Print and shaded views of the part. All mm, measured from the part's lowest x, y and z. A direction names the side the tool comes from. Round coordinates to 2 decimals unless told otherwise and drop trailing zeros. Write each loop counter-clockwise with the first axis right and the second up, starting at its lowest first coordinate (ties: lowest second). Pieces come first, ordered by that corner, then holes. Notation, with made-up numbers: (42, -30.75) - (77, -30.75) arc R13 cw to (77, -9.75) - close; hole circle Ø2 at (60.5, 6.25). An arc over 180 degrees is marked (long way). Answer as a JSON object with one key per item and string values. Group by question number.
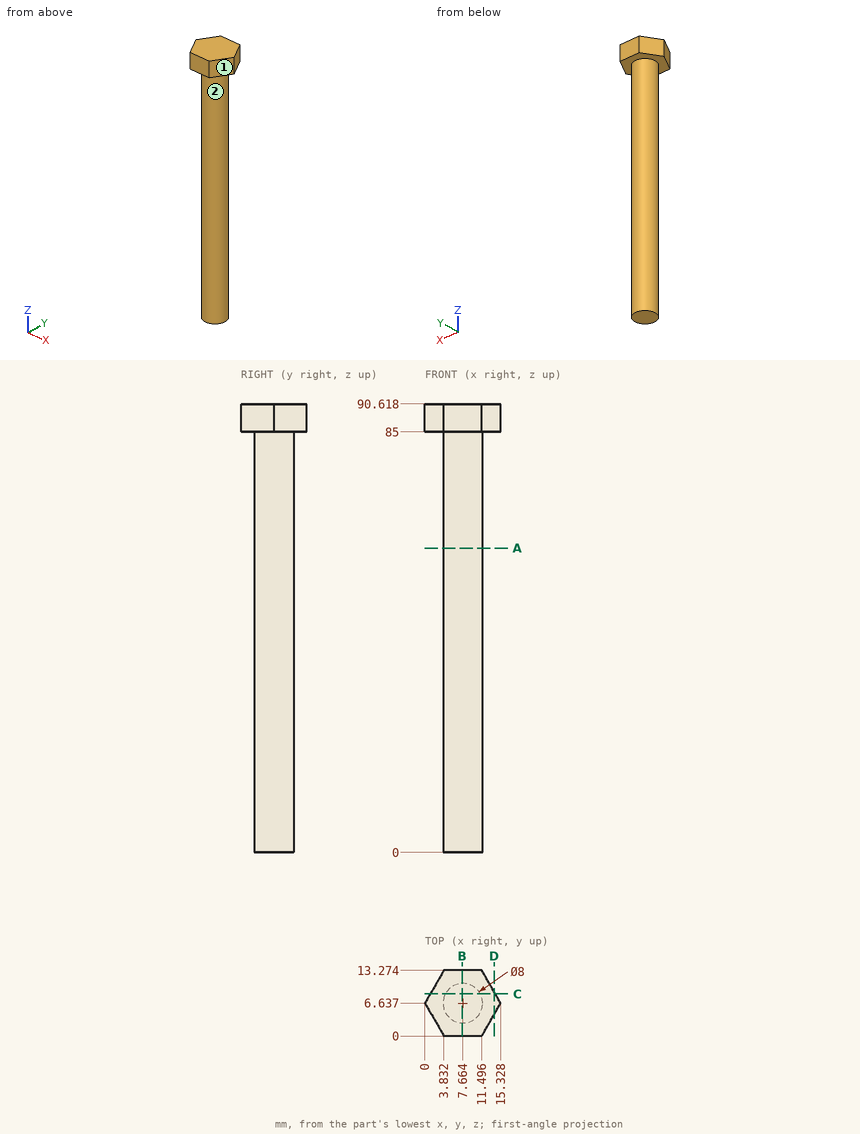
(1) 3-axis set-ups, long thin cutter, end or side, ignore diameter. For the marked faces 1 and 2: which of +Z, -Z, +X, -X, +Y, -Y reach the whole face in a straight line?
(2) Flat gauge pins, fed straight in: pin 1 (4 mm diameter, centred on x = 11, z = 34.5, fed in from +Y); pin 2 (5 mm diameter, centred on y = 3.5, z = 30.5, fed in from +X); pin 3 (4 mm diameter, centred on x = 6, y = 4.5, fed in from -Z); pin 4 (4 mm diameter, centred on x = 2.5, z = 35.5, fed in from +Y) (1 decimal). Where does each tip first touch, or does it go through?
(3) Slice it at B-B (x = 7.5). Write the cut outline in (y, z) (1 decimal), then the cut area to 3 significant figures.
(4) Slice it at C-C (y = 8.5). Write the cut outline in (x, z) (1 decimal), then the cut area to 3 significant figures.
(5) Slice it at A-A (z = 61.5). Write the cut outline in (x, y) (1 decimal).
(6) Slice it at D-D (x = 14). Write the cut outline in (y, z).
(7) Drill centre lines: line 1 (Z direction, x = 11.75, y = 9); line 2 (X direction, y = 6.5, z = 84); line 3 (Y direction, x = 8, z = 74). Where is each one in solid material? Low to high. Write a range as from..to.
Answer:
{
 "1": {"face 1": "+Z, -Z, +X, -Y", "face 2": "-Z"},
 "2": {"pin 1": "y = 10.41", "pin 2": "x = 11.61", "pin 3": "z = 0", "pin 4": "y = 9.1"},
 "3": {"outline": "(0, 85) - (2.6, 85) - (2.6, 0) - (10.6, 0) - (10.6, 85) - (13.3, 85) - (13.3, 90.6) - (0, 90.6) - close", "area": "754 mm²"},
 "4": {"outline": "(1.1, 85) - (4.1, 85) - (4.1, 0) - (11.2, 0) - (11.2, 85) - (14.3, 85) - (14.3, 90.6) - (1.1, 90.6) - close", "area": "676 mm²"},
 "5": {"outline": "circle Ø8 at (7.7, 6.6)"},
 "6": {"outline": "(4.34, 85) - (8.94, 85) - (8.94, 90.62) - (4.34, 90.62) - close"},
 "7": {"line 1": "85..90.62", "line 2": "3.67..11.66", "line 3": "2.65..10.62"}
}
